from build123d import *

# Parameters (mm, degrees)
SKETCH025_W     = 45
SKETCH025_H     = 65
PAD010_DEPTH    = 110
FILLET009_R     = 6
SKETCH026_W     = 30
SKETCH026_H     = 92
POCKET013_DEPTH = 12
SKETCH027_R     = 2
PAD011_DEPTH    = 10
SKETCH028_W     = 65
SKETCH028_H     = 50
POCKET014_DEPTH = 5
FILLET010_R     = 20
FILLET011_R     = 3


with BuildPart() as part:
    # Sketch025 → Pad010 (new body)
    with BuildSketch(Plane.XY):
        Rectangle(SKETCH025_W, SKETCH025_H)
    extrude(amount=PAD010_DEPTH)

    # Fillet009
    fillet009_edges = [part.edges().sort_by_distance(p)[0] for p in [
        (-22.5, 0, 110),
        (22.5, 0, 110),
    ]]
    fillet(fillet009_edges, radius=FILLET009_R)

    # Sketch026 (on Face2 of Fillet009) → Pocket013 (cut)
    with BuildSketch(Plane.XZ.offset(32.5)):
        with Locations((2.5, 59)):
            Rectangle(SKETCH026_W, SKETCH026_H)
    pocket013 = extrude(amount=-POCKET013_DEPTH, mode=Mode.SUBTRACT)

    # Mirrored001: Pocket013 across XZ
    add(pocket013.mirror(Plane.XZ), mode=Mode.SUBTRACT)

    # Sketch027 (on Face17 of Mirrored001) → Pad011 (join)
    with BuildSketch(Plane.XZ.offset(20.5)):
        with Locations((-5, 101)):
            Circle(SKETCH027_R)
        with Locations((10, 101)):
            Circle(SKETCH027_R)
    extrude(amount=PAD011_DEPTH)

    # Sketch028 (on Face1 of Pad011) → Pocket014 (cut)
    with BuildSketch(Plane(origin=(-22.5, 0, 0), x_dir=(0, -1, 0), z_dir=(-1, 0, 0))):
        with Locations((0, 25)):
            Rectangle(SKETCH028_W, SKETCH028_H)
    extrude(amount=-POCKET014_DEPTH, mode=Mode.SUBTRACT)

    # Fillet010
    fillet010_edges = [part.edges().sort_by_distance(p)[0] for p in [
        (-20, 32.5, 50),
        (-20, -32.5, 50),
    ]]
    fillet(fillet010_edges, radius=FILLET010_R)

    # Fillet011
    fillet011_edges = [part.edges().sort_by_distance(p)[0] for p in [
        (-17.5, 0, 0),
        (22.5, 0, 0),
    ]]
    fillet(fillet011_edges, radius=FILLET011_R)


solid = part.part
Could you check a few things on this model? Use its own coordinates, in mm. A direction names the side the tool comes from. Give positions to 0.01 mm unless a question says otherwise; leave off trailing zeros. Order: outer loops, then holes, each group sorted by start corner. A loop starts at its lowest first (then second) coordinate and runs counter-clockwise, first axis right, second up. Notation, with made-up numbers: (-7, -6) -> (0, -6) arc R22 cw to (0, 20) -> close; hole circle Ø2 at (44.5, 17.5). An arc over 180 degrees is marked (long way). Answer in a Markdown table with one row per item. Add a question column.
Item 1: I'm going to push flat-ended pins straight in: P1, Ø4.5, axis at x = 11, z = 101, coming from the -Y side; P2, Ø4, axis at x = -16.5, y = 9, coming from the -Z side; P3, Ø1.5, axis at x = -19, y = -3, coming from the -Z side; P4, Ø6, axis at y = -25, z = 44, coming from the -X side. Where does each tip first touch, or does it pass through?
Item 2: Imagine slicing it at D-D (y = -25.5). List the corners of the cut face in (x, z) for me, and give its area (3 significant figures).
Item 3: Imagine slicing it at C-C (x = 10). List the corners of the cut face in (y, z) for me.
Item 4: Imagine slicing it at A-A (y = 28.5). List the corners of the cut face in (x, z) for me, and give its area (3 significant figures).
Item 5: Imagine slicing it at B-B (z = 91.5). List the corners of the cut face in (x, y) for me, and give its area (4 significant figures).
Item 6: For faces 1 (the flat face through (2, 27, 13)), 2 (the flat face through (2, 0, 0)), 3 (the cylindrical face through (-19.965, 26.486, 55.703)), 4 (the cylindrical face through (-16.6, -0.45, 0.86)), 5 (the flat face through (-12.5, -27, 58)), which set-ups out of +Z, -Z, +X, -X, +Y, -Y let a thin tool reach every point of the face, with its end or its side?
Item 7: We'd pull the mould along X, two halves only. Please class faces 6 (the cylindrical face through (-19.965, -26.486, 55.703)), 7 (the flat face through (2, -27, 13)), 8 (the cylindrical face through (20.789, 0.455, 108.196)): pulls with the +X half, pulls with the -X half, needs draft (parallel to the pull), parting line crosses it, or undercut.
Item 8: Please list where these lines run through material, in increasing order: probe 1 along Z at (x, y) = (11.5, 26); probe 2 along Z at (x, y) = (10, -28.5); probe 3 along X at (y, z) = (22, 14.5).
Result:
| question | item | result |
|---|---|---|
| 1 | P1 | y = -30.5 |
| 1 | P2 | z = 0 |
| 1 | P3 | z = 50 |
| 1 | P4 | x = -17.5 |
| 2 | outline | (-22.5, 54.8) -> (-17.5, 54.8) -> (-17.5, 3) arc R3 ccw to (-14.5, 0) -> (19.5, 0) arc R3 ccw to (22.5, 3) -> (22.5, 104) arc R6 ccw to (16.5, 110) -> (-16.5, 110) arc R6 ccw to (-22.5, 104) -> close; circle Ø4 at (-5, 101); circle Ø4 at (10, 101); hole (-12.5, 13) -> (17.5, 13) -> (17.5, 105) -> (-12.5, 105) -> close |
| 2 | area | 1,920 mm2 |
| 3 | outline | (-32.5, 0) -> (32.5, 0) -> (32.5, 13) -> (20.5, 13) -> (20.5, 105) -> (32.5, 105) -> (32.5, 110) -> (-32.5, 110) -> (-32.5, 105) -> (-20.5, 105) -> (-20.5, 103) -> (-30.5, 103) -> (-30.5, 99) -> (-20.5, 99) -> (-20.5, 13) -> (-32.5, 13) -> close |
| 4 | outline | (-22.5, 58) -> (-17.5, 58) -> (-17.5, 3) arc R3 ccw to (-14.5, 0) -> (19.5, 0) arc R3 ccw to (22.5, 3) -> (22.5, 104) arc R6 ccw to (16.5, 110) -> (-16.5, 110) arc R6 ccw to (-22.5, 104) -> close; hole (-12.5, 13) -> (17.5, 13) -> (17.5, 105) -> (-12.5, 105) -> close |
| 4 | area | 1,880 mm2 |
| 5 | outline | (-22.5, -32.5) -> (-12.5, -32.5) -> (-12.5, -20.5) -> (17.5, -20.5) -> (17.5, -32.5) -> (22.5, -32.5) -> (22.5, 32.5) -> (17.5, 32.5) -> (17.5, 20.5) -> (-12.5, 20.5) -> (-12.5, 32.5) -> (-22.5, 32.5) -> close |
| 5 | area | 2,205 mm2 |
| 6 | face 1 | +Y |
| 6 | face 2 | -Z, +X, -X, +Y, -Y |
| 6 | face 3 | -Z, -X, +Y |
| 6 | face 4 | -Z, -X, +Y, -Y |
| 6 | face 5 | -Y |
| 7 | face 6 | needs draft |
| 7 | face 7 | undercut |
| 7 | face 8 | pulls with the +X half |
| 8 | probe 1 | 0 to 13, 105 to 110 |
| 8 | probe 2 | 0 to 13, 99 to 103, 105 to 110 |
| 8 | probe 3 | -17.5 to -12.5, 17.5 to 22.5 |
